Answer from the drawing. Dimensions are ordinates in mm from the lowest x, y and z of the part. Give positions to 0.01 mm unless a question says otherwise; leave off trailing zeros. Loops run counter-clockwise (first coordinate to the right, second up) from the corner with the lowest first, then second, coordinate; pieces in that order, holes last. Notation, with made-up numbers: M -19.5,-32 L 14.5,-32 A28 cw 14.5,-11 Z; hole C -4.5,17 d4. An arc over 180 degrees is marked long. Use a Markdown table: item, result.
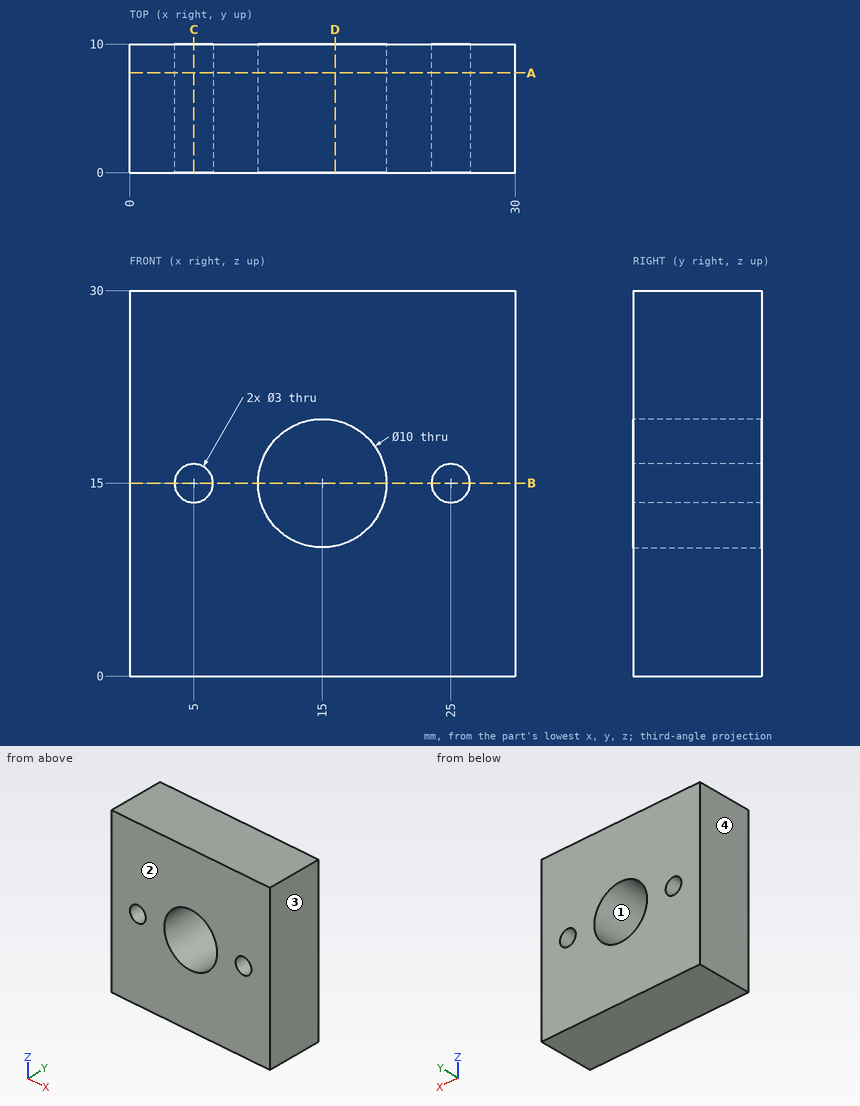
(1) Consider probe 1 along X at (y, z) = (2.25, 15); probe 2 along Z at (x, y) = (5, 2.75); probe 3 along X at (y, z) = (5.25, 15.75). Determine where each line is inside the solid, lowest interval first. Write a range as [from, to].
Entries:
| item | result |
|---|---|
| probe 1 | x = [0, 3.5], [6.5, 10], [20, 23.5], [26.5, 30] |
| probe 2 | z = [0, 13.5], [16.5, 30] |
| probe 3 | x = [0, 3.7], [6.3, 10.06], [19.94, 23.7], [26.3, 30] |
(2) The mould has two halves that part along X. Classify the marked faces 1, 2, 3 and 4: released by +X, released by -X, zero draft, split by the parting line, or undercut.
Entries:
| item | result |
|---|---|
| face 1 | undercut |
| face 2 | zero draft |
| face 3 | released by +X |
| face 4 | released by -X |
(3) A cutting plane is placed at B-B (z = 15). Write down the section's boundary in (x, y), and give its area (3 significant figures).
Entries:
| item | result |
|---|---|
| outline | M 0,0 L 3.5,0 L 3.5,10 L 0,10 Z; M 6.5,0 L 10,0 L 10,10 L 6.5,10 Z; M 20,0 L 23.5,0 L 23.5,10 L 20,10 Z; M 26.5,0 L 30,0 L 30,10 L 26.5,10 Z |
| area | 140 mm² |
(4) A cutting plane is placed at A-A (y = 7.75). Write down the section's boundary in (x, z), and give its area (3 significant figures).
Entries:
| item | result |
|---|---|
| outline | M 0,0 L 30,0 L 30,30 L 0,30 Z; hole C 5,15 d3; hole C 15,15 d10; hole C 25,15 d3 |
| area | 807 mm² |
(5) Given P1, Ø8, axis at x = 15, z = 15, coming from the -Y side (3 decimals), flat-ended and moving along its own axis, determine where the tip first touches the part or whether it passes through.
Entries:
| item | result |
|---|---|
| P1 | passes through |
(6) A cutting plane is placed at C-C (x = 5). Write down the section's boundary in (y, z).
Entries:
| item | result |
|---|---|
| outline | M 0,0 L 10,0 L 10,13.5 L 0,13.5 Z; M 0,16.5 L 10,16.5 L 10,30 L 0,30 Z |
(7) A cutting plane is placed at D-D (x = 16). Write down the section's boundary in (y, z).
Entries:
| item | result |
|---|---|
| outline | M 0,0 L 10,0 L 10,10.1 L 0,10.1 Z; M 0,19.9 L 10,19.9 L 10,30 L 0,30 Z |
